The drawing under review shows one solid part. Ordinate dimensions are in mm from its lowest x, y, z. A direction names the side the tool comes from. Round coordinates to 2 decimals unless told otherwise and drop trailing zeros. Write each loop counter-clockwise with the first axis right and the second up, starting at its lowest first coordinate (ties: lowest second). Pieces come first, ordered by that corner, then holes. Notation, with made-up numbers: (-7.75, 78.5) -> (13.25, 78.5) arc R21 cw to (13.25, 92.5) -> close; hole circle Ø7 at (-17.5, 36.25). An arc over 180 degrees is marked (long way). Answer in a Markdown table with one row per item.
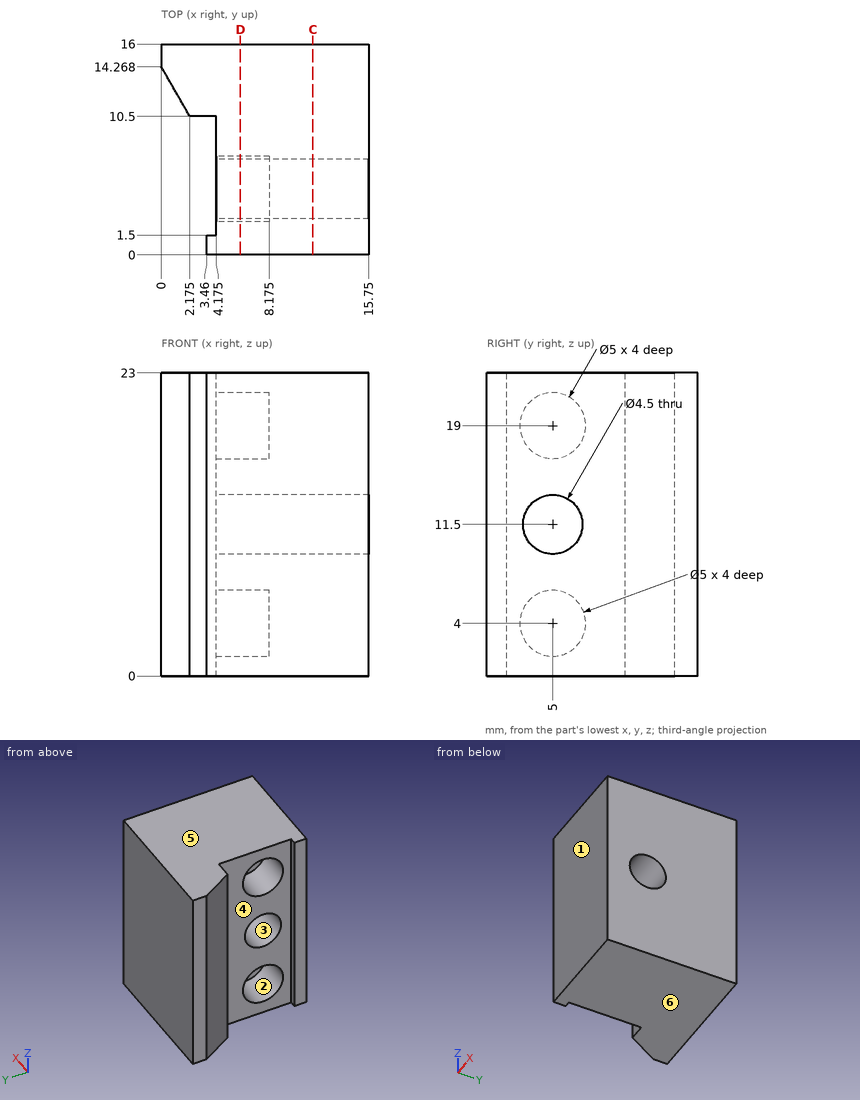
1) Consider section D-D on x = 6. State the section outline as (y, z) points, then the cut area to 3 significant figures.
Solved:
| item | result |
|---|---|
| outline | (0, 0) -> (16, 0) -> (16, 23) -> (0, 23) -> close; hole circle Ø5 at (5, 4); hole circle Ø5 at (5, 19); hole circle Ø4.5 at (5, 11.5) |
| area | 313 mm² |
2) Consider section C-C on x = 11.5. State the section outline as (y, z) points, then the cut area to 3 significant figures.
Solved:
| item | result |
|---|---|
| outline | (0, 0) -> (16, 0) -> (16, 23) -> (0, 23) -> close; hole circle Ø4.5 at (5, 11.5) |
| area | 352 mm² |
3) Mouldability with a two-part tool opening along Z and no side actions: class the marked faces 3, 4, 5 and 6 as pulls with the +Z half, pulls with the -Z half, needs draft (parallel to the pull), parting line crosses it, or undercut.
Solved:
| item | result |
|---|---|
| face 3 | undercut |
| face 4 | needs draft |
| face 5 | pulls with the +Z half |
| face 6 | pulls with the -Z half |
4) For the marked faces 1 and 2, list the 3-axis set-ups (+Z, -Z, +X, -X, +Y, -Y) from which the entire face can be reached by the end or side of a thin tool; tool diameter is ignored.
Solved:
| item | result |
|---|---|
| face 1 | +Z, -Z, +X, -X, -Y |
| face 2 | -X |
5) For line 1 (Y direction, x = 3.5, z = 12); line 2 (Z direction, x = 7.5, y = 7) (1 decimal); line 3 (Y direction, x = 5.05, z = 19), list the stretches that pass through material, from the lowest coordinate up. Write a range as [from, to].
Solved:
| item | result |
|---|---|
| line 1 | [0, 1.5], [10.5, 16] |
| line 2 | [0, 2.5], [5.5, 10.5], [12.5, 17.5], [20.5, 23] |
| line 3 | [0, 2.5], [7.5, 16] |
6) Clearance check with flat-ended pins moving along their axes: pin 1 Ø1.5 at (y, z) = (5, 18) entering from -X (1 decimal); pin 2 Ø4.5 at (y, z) = (4.5, 9) entering from -X (1 decimal). State where each tip first meets the part, or that it passes through.
Solved:
| item | result |
|---|---|
| pin 1 | x = 8.2 |
| pin 2 | x = 4.2 |
